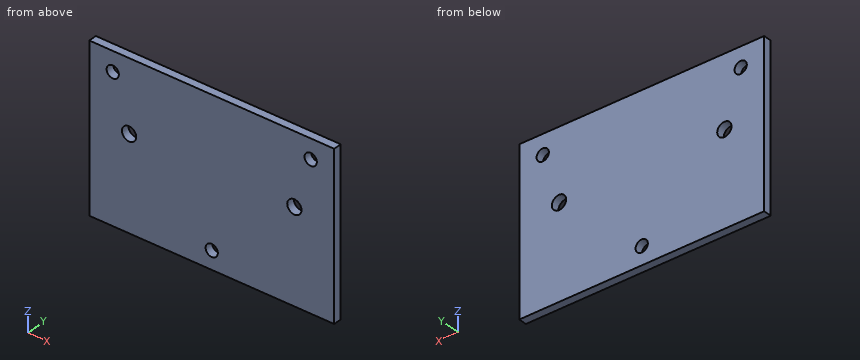
Autodesk Inventor part; units mm, degrees
ref_plane "YZ Plane" through (0, 0, 0) normal (1, 0, 0) x (0, 1, 0)
ref_plane "XZ Plane" through (0, 0, 0) normal (0, 1, 0) x (-1, 0, 0)
ref_plane "XY Plane" through (0, 0, 0) normal (0, 0, 1) x (1, 0, 0)
sketch "Szkic1" plane through (0, 0, 0) normal (0, 1, 0) x (-1, 0, 0)
  line L0 (-75.7688, 32.9192) -> (-75.7688, 6.9192)
  line L1 (-75.7688, 6.9192) -> (-15.7688, 6.9192)
  line L2 (-15.7688, 6.9192) -> (-15.7688, 32.9192)
  circle A0 centre (-70.0174, 42.1278) radius 1.5
  circle A1 centre (-21.5202, 42.1278) radius 1.5
  circle A2 centre (-45.7688, 11.3479) radius 1.5
  circle A3 centre (-25.5188, 29.6192) radius 1.75
  circle A4 centre (-66.0188, 29.6192) radius 1.75
  line L3 (-75.7688, 6.9192) -> (-15.7688, 6.9192)
  line L4 (-15.7688, 6.9192) -> (-15.7688, 46.9192)
  line L5 (-15.7688, 46.9192) -> (-75.7688, 46.9192)
  line L6 (-75.7688, 46.9192) -> (-75.7688, 6.9192)
  point P0 (0, 0)
  dimension "d0" = 40
extrude "Wyciągnięcie proste1" add sketch "Szkic1" along normal blind 2
properties part number "dociazenie"
Here's how the part is built. I have some questions about the finished solid (model axes, mm). Round coordinates to 2 decimals unless told otherwise and drop trailing zeros. Loops run counter-clockwise (first coordinate to the right, second up) from the corner with the lowest first, then second, coordinate; pieces in that order, holes last. Notation, with made-up numbers: (48.5, 42) -> (60.5, 42) arc R18 cw to (60.5, 57) -> close; hole circle Ø4 at (-13, 80). An arc over 180 degrees is marked (long way). Write each question's results on one line, items separated by ' | '.
(1) If we section it at C-C, the plane x = 66: List the corners of the cut face in (y, z) for me, then the cut area to 3 significant figures.
Worked answers:
outline: (0, 6.92) -> (2, 6.92) -> (2, 27.87) -> (0, 27.87) -> close; (0, 31.37) -> (2, 31.37) -> (2, 46.92) -> (0, 46.92) -> close | area: 73.0 mm2
(2) If we section it at B-B, the plane y = 0.4: List the corners of the cut face in (x, z) for me, then the cut area to 3 significant figures.
Worked answers:
outline: (15.77, 6.92) -> (75.77, 6.92) -> (75.77, 46.92) -> (15.77, 46.92) -> close; hole circle Ø3 at (21.52, 42.13); hole circle Ø3.5 at (25.52, 29.62); hole circle Ø3 at (45.77, 11.35); hole circle Ø3.5 at (66.02, 29.62); hole circle Ø3 at (70.02, 42.13) | area: 2,360 mm2
(3) If I drill on L1, parallel to X at y = 1.85, z = 42; L2, parallel to X at y = 0.7, z = 11.5; L3, parallel to X at y = 0.9, z = 43.5, over which ranges is the centre line in solid material (lowest first)?
Worked answers:
L1: 15.77 to 20.03, 23.01 to 68.52, 71.51 to 75.77 | L2: 15.77 to 44.28, 47.26 to 75.77 | L3: 15.77 to 20.91, 22.13 to 69.41, 70.62 to 75.77
(4) If we section it at A-A, the plane x = 22: List the corners of the cut face in (y, z) for me.
Worked answers:
outline: (0, 6.92) -> (2, 6.92) -> (2, 40.71) -> (0, 40.71) -> close; (0, 43.55) -> (2, 43.55) -> (2, 46.92) -> (0, 46.92) -> close
